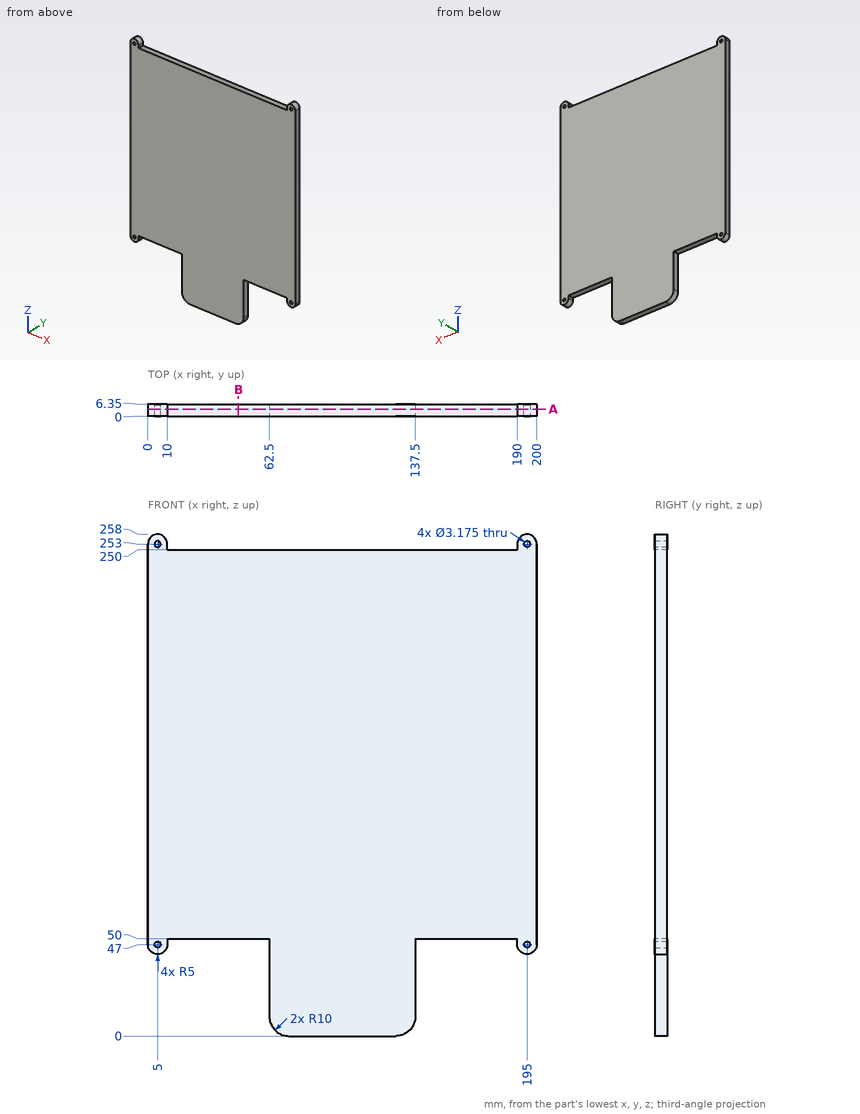
Input: dimensioned drawing with shaded views. Units: mm. Origin: part minimum x, y, z. Round coordinates to 2 decimals unless told otherwise and drop trailing zeros. Order: outer loops, then holes, each group sorted by start corner. A loop starts at its lowest first (then second) coordinate and runs counter-clockwise, first axis right, second up. Notation, with made-up numbers: M -32,51 L 21,51 A16 ccw 21,75 Z; hole C 29.5,85.5 d5. An arc over 180 degrees is marked long. Use one line per item in the form item = value. Start each with the question number.
Q1. Pin query (flat end, axial travel): pin 1 Ø3 at (x, y) = (165, 4) entering from -Z; pin 2 Ø3 at (x, y) = (87.5, 3) entering from +Z; pin 3 Ø1.5 at (x, y) = (129.5, 5.5) entering from -Z; pin 4 Ø3 at (x, z) = (195, 47) entering from -Y. Return the tip coordinate at first contact, or that it passes through.
Q2. Cut plane A-A (y = 3.75). Return loops of the section in (x, z) (1 decimal).
Q3. Material intervals for line 1 (X direction, y = 4, z = 253); line 2 (Z direction, x = 5, y = 4.5); line 3 (X direction, y = 5, z = 47), sorted ascending. Write a range as [from, to].
Q4. Cut plane B-B (x = 46.5). Return loops of the section in (y, z), and give its area (3 significant figures).
Geometry results:
q1.pin_1 = 50
q1.pin_2 = 250
q1.pin_3 = 0.08
q1.pin_4 = through
q2.outline = M 0,47 A5 ccw 10,47 L 10,50 L 62.5,50 L 62.5,10 A10 ccw 72.5,0 L 127.5,0 A10 ccw 137.5,10 L 137.5,50 L 190,50 L 190,47 A5 ccw 200,47 L 200,253 A5 ccw 190,253 L 190,250 L 10,250 L 10,253 A5 ccw 0,253 Z; hole C 5,47 d3.2; hole C 5,253 d3.2; hole C 195,47 d3.2; hole C 195,253 d3.2
q3.line_1 = [0, 3.41], [6.59, 10], [190, 193.41], [196.59, 200]
q3.line_2 = [42, 45.41], [48.59, 251.41], [254.59, 258]
q3.line_3 = [0, 3.41], [6.59, 10], [62.5, 137.5], [190, 193.41], [196.59, 200]
q4.outline = M 0,50 L 6.35,50 L 6.35,250 L 0,250 Z
q4.area = 1,270 mm^2
